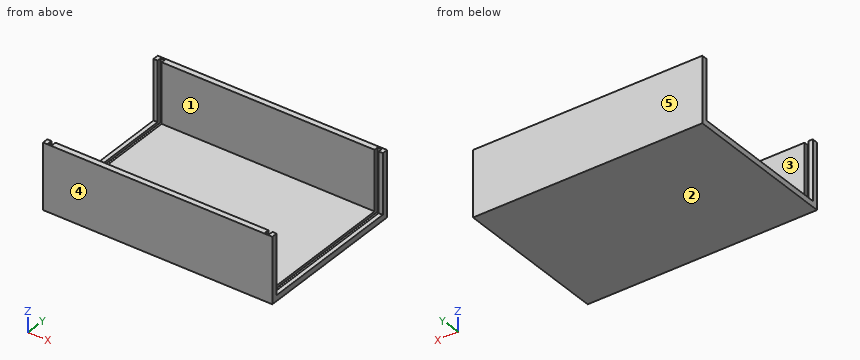
```python
from build123d import *

# Parameters (mm, degrees)
SKETCH001_W     = 140
SKETCH001_H     = 95
PAD002_DEPTH    = 3.5
SKETCH006_W     = 140
SKETCH006_H     = 3.5
PAD003_DEPTH    = 36.5
SKETCH007_W     = 2.5
SKETCH007_H     = 93
POCKET001_DEPTH = 38


with BuildPart() as part:
    # Sketch001 → Pad002 (new body)
    with BuildSketch(Plane.XY):
        Rectangle(SKETCH001_W, SKETCH001_H)
    extrude(amount=-PAD002_DEPTH)

    # Sketch006 → Pad003 (join)
    with BuildSketch(Plane.XY):
        with Locations((0, 45.75)):
            Rectangle(SKETCH006_W, SKETCH006_H)
        with Locations((0, -45.75)):
            Rectangle(SKETCH006_W, SKETCH006_H)
    extrude(amount=PAD003_DEPTH)

    # Sketch007 (on Face16 of Pad003) → Pocket001 (cut)
    with BuildSketch(Plane.XY.offset(36.5)):
        with Locations((-66.25, 0)):
            Rectangle(SKETCH007_W, SKETCH007_H)
        with Locations((66.25, 0)):
            Rectangle(SKETCH007_W, SKETCH007_H)
    extrude(amount=-POCKET001_DEPTH, mode=Mode.SUBTRACT)


solid = part.part
```
For this review, take the finished solid that the model builds, in its own axes (mm). Face numbers are marked on the shaded views. A direction names the side the tool comes from. Give positions to 0.01 mm unless a question says otherwise; leave off trailing zeros. Write each loop counter-clockwise with the first axis right and the second up, starting at its lowest first coordinate (ties: lowest second). Pieces come first, ordered by that corner, then holes. Notation, with made-up numbers: M 20,26 L 77,26 A20 cw 77,49 Z; hole C 87,-3 d10. An arc over 180 degrees is marked long. One line per item, written item: value.
1) The part is to be moulded in two halves that separate along Y. For the marked faces 3, 4 and 5, say which applies: +Y half, -Y half, draft (parallel to the pull), parting line (faces both ways), or undercut.
Results are:
face 3: undercut
face 4: -Y half
face 5: +Y half
2) For the marked faces 1 and 2, list the 3-axis set-ups (+Z, -Z, +X, -X, +Y, -Y) from which the entire face can be reached by the end or side of a thin tool; tool diameter is ignored.
Results are:
face 1: +Z, +X, -X
face 2: -Z, +X, -X, +Y, -Y
3) Take a section at C-C, the plane x = 20. Write out the cut boundary in (y, z).
Results are:
outline: M -47.5,-3.5 L 47.5,-3.5 L 47.5,36.5 L 44,36.5 L 44,0 L -44,0 L -44,36.5 L -47.5,36.5 Z
4) Take a section at A-A, the plane z = 18.5. Write out the cut boundary in (x, y).
Results are:
outline: M -70,-47.5 L 70,-47.5 L 70,-44 L 67.5,-44 L 67.5,-46.5 L 65,-46.5 L 65,-44 L -65,-44 L -65,-46.5 L -67.5,-46.5 L -67.5,-44 L -70,-44 Z; M -70,44 L -67.5,44 L -67.5,46.5 L -65,46.5 L -65,44 L 65,44 L 65,46.5 L 67.5,46.5 L 67.5,44 L 70,44 L 70,47.5 L -70,47.5 Z
5) For P1, Ø10, axis at x = -52, y = 28, coming from the +Z side; P2, Ø0.8, axis at x = -66, y = -11.5, coming from the +Z side, all flat-tipped, find the tip position at first contact; note any pin that passes through.
Results are:
P1: stops at z = 0
P2: stops at z = -1.5
6) For line 1 (Y direction, x = -14.5, z = 21); line 2 (Z direction, x = 25, y = 32.5), list the stretches that pass through material, from the lowest coordinate up. Write a range as from..to.
Results are:
line 1: y = -47.5..-44, 44..47.5
line 2: z = -3.5..0
7) Take a section at B-B, the plane y = -6. Write out the cut boundary in (x, z).
Results are:
outline: M -70,-3.5 L 70,-3.5 L 70,0 L 67.5,0 L 67.5,-1.5 L 65,-1.5 L 65,0 L -65,0 L -65,-1.5 L -67.5,-1.5 L -67.5,0 L -70,0 Z
